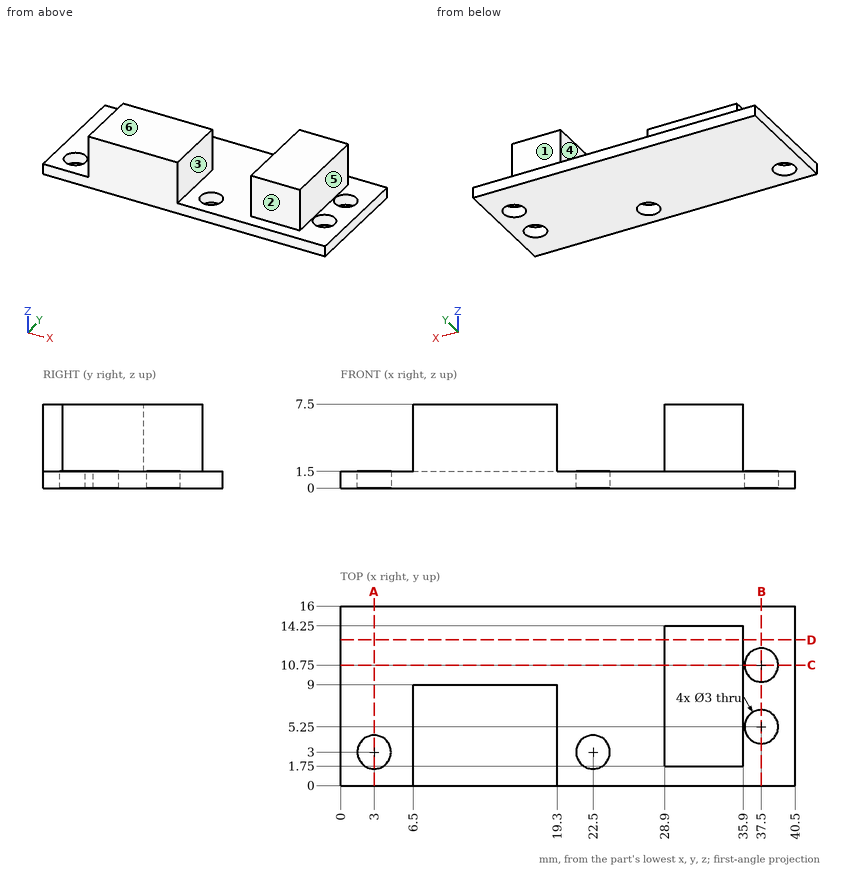
Study the drawing (mm; zero at the part's minimum x, y, z) and answer. A direction names the side the tool comes from. Coordinates: 2 decimals unless noted, no trailing zeros. Loops run counter-clockwise (first coordinate to the right, second up) from the corner with the lowest first, then second, coordinate; pieces in that order, holes last. Notation, with made-up numbers: M -15.5,-38.75 L 20.5,-38.75 A33 cw 20.5,-4.75 Z; hole C 78,40.5 d5. An arc over 180 degrees is marked long. Answer in a Markdown table with one row per item. Add a question column.
1. Consider L1, parallel to Y at x = 37.5, z = 0.9; L2, parallel to Y at x = 3, z = 0.5; L3, parallel to X at y = 4.75, z = 5.75. Determine where each line is inside the solid, lowest interval first.
2. Find section D-D, the plane y = 13. Write down the section's boundary in (x, z).
3. The mould has two halves that part along X. Classify the marked faces 4, 5 and 6: pulls with the +X half, pulls with the -X half, needs draft (parallel to the pull), parting line crosses it, or undercut.
4. Find section B-B, the plane x = 37.5. Write down the section's boundary in (y, z), then the cut area to 3 significant figures.
5. Find section A-A, the plane x = 3. Write down the section's boundary in (y, z), then the cut area to 3 significant figures.
6. A tool of negligible diameter and unlimited length cuts with its end or side. For the marked faces 1, 2 and 3, from which of +Z, -Z, +X, -X, +Y, -Y can it reach the whole face along a straight path? Write none if from no direction.
7. Find section C-C, the plane y = 10.75. Write down the section's boundary in (x, z).
8. Flat-ended cylindrical pins translate along their axes: P1, Ø4, axis at x = 37.5, y = 10.75, coming from the +Z side; P2, Ø1, axis at x = 11.5, z = 5.5, coming from the +Y side; P3, Ø1.8, axis at y = 6, z = 3.5, coming from the -X side; P4, Ø3, axis at y = 11, z = 4.5, coming from the -X side. Find the tip coordinate at first contact, or state that the pin passes through.
Reported:
| question | item | result |
|---|---|---|
| 1 | L1 | y = 0 to 3.75, 6.75 to 9.25, 12.25 to 16 |
| 1 | L2 | y = 0 to 1.5, 4.5 to 16 |
| 1 | L3 | x = 6.5 to 19.3, 28.9 to 35.9 |
| 2 | outline | M 0,0 L 40.5,0 L 40.5,1.5 L 35.9,1.5 L 35.9,7.5 L 28.9,7.5 L 28.9,1.5 L 0,1.5 Z |
| 3 | face 4 | undercut |
| 3 | face 5 | pulls with the +X half |
| 3 | face 6 | needs draft |
| 4 | outline | M 0,0 L 3.75,0 L 3.75,1.5 L 0,1.5 Z; M 6.75,0 L 9.25,0 L 9.25,1.5 L 6.75,1.5 Z; M 12.25,0 L 16,0 L 16,1.5 L 12.25,1.5 Z |
| 4 | area | 15.0 mm^2 |
| 5 | outline | M 0,0 L 1.5,0 L 1.5,1.5 L 0,1.5 Z; M 4.5,0 L 16,0 L 16,1.5 L 4.5,1.5 Z |
| 5 | area | 19.5 mm^2 |
| 6 | face 1 | +Z, +X, -X, +Y |
| 6 | face 2 | +Z, +X, -Y |
| 6 | face 3 | +Z, +Y, -Y |
| 7 | outline | M 0,0 L 36,0 L 36,1.5 L 35.9,1.5 L 35.9,7.5 L 28.9,7.5 L 28.9,1.5 L 0,1.5 Z; M 39,0 L 40.5,0 L 40.5,1.5 L 39,1.5 Z |
| 8 | P1 | stops at z = 7.5 |
| 8 | P2 | stops at y = 9 |
| 8 | P3 | stops at x = 6.5 |
| 8 | P4 | stops at x = 28.9 |
